Verification items for the finished model (mm, model axes). Face numbers are marked on the shaded views. A direction names the side the tool comes from. Give positions to 0.01 mm unless a question says otherwise; leave off trailing zeros. Order: outer loops, then holes, each group sorted by start corner. A loop starts at its lowest first (then second) coordinate and runs counter-clockwise, first axis right, second up. Notation, with made-up numbers: (65, -19) -> (77, -19) arc R36 ccw to (77, 16) -> close; hole circle Ø10 at (11, 72.25). An arc over 180 degrees is marked (long way). Return JSON: item names as keys, results as strings. Group by question number.
(1) Depth check by flat-ended pin: pin 1 Ø1 at (x, z) = (1, 2.5) entering from -Y; pin 2 Ø5 at (y, z) = (0.5, -9) entering from +X; pin 3 Ø2 at (x, z) = (-1, -8.5) entering from +Y. Enter the tip coordinate at first touch or a pass-through.
(2) Cross-section at B-B on z = -11.5. Enter the section's corners in (x, y), then the cut area to 3 significant figures.
(3) Thickness scan on line 1 along Z through (x, y) = (2.25, -2.25); line 2 along X through (y, z) = (1.75, -12.75); line 3 along Z through (x, y) = (0.25, -0.5). Record the ranges inside material, lowest first.
(4) Release check for a two-part mould opening along X. For the marked faces 3, 4 and 5 record: pulls with the +X half, pulls with the -X half, needs draft (parallel to the pull), parting line crosses it, or undercut.
(5) Tool access check on the marked faces 1 and 2. Record the directions out of +Z, -Z, +X, -X, +Y, -Y that give a thin tool (end or side, any length) a straight path to the whole face; none if there is none.
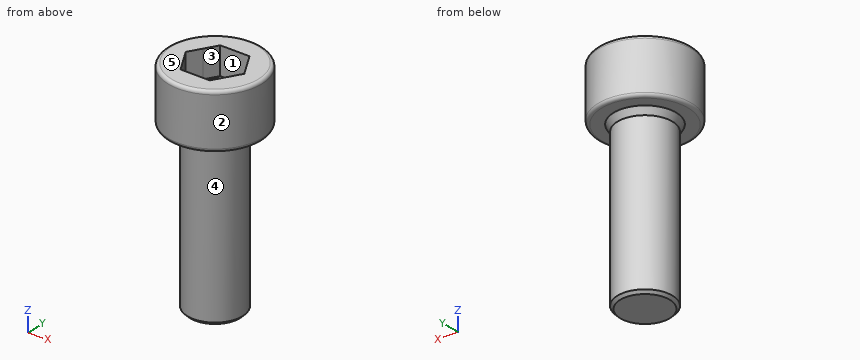
Solid Edge part; units mm, degrees
sketch "Sketch1" plane through (0, 0, 0) normal (0, -1, 0) x (1, 0, 0)
  line L0 (4.25, 5) -> (4.25, 0)
  line L1 (4.25, 0) -> (2.85, 0)
  line L2 (2.85, 0) -> (2.5, -0.6062)
  line L3 (2.5, -0.6062) -> (2.5, -15)
  line L4 (2.5, -15) -> (0, -15)
  line L5 (2.3, 2.5) -> (0, 1.1721)
  line L6 (2.3, 5) -> (2.3, 2.5)
  line L7 (4.25, 5) -> (2.3, 5)
revolve "RevolvedProtrusion1" add sketch "Sketch1" angle 360 about axis through (0, 0, -6) along (0, 0, 1)
cosmetic_thread "Thread1"
chamfer "chamfer" distance 0.25 angle 45 1 edges at (-2.5, 0, -15)
fillet "head_roundings" radius 0.3 2 edges at (-4.25, 0, 0) (-4.25, 0, 5)
sketch "Sketch2" plane through (0, 0, 5) normal (0, 0, 1) x (0, 1, 0)
  line L0 (-2.3, 1.3279) -> (-2.3, -1.3279)
  line L1 (0, -2.6558) -> (-2.3, -1.3279)
  line L2 (2.3, -1.3279) -> (0, -2.6558)
  line L3 (2.3, 1.3279) -> (2.3, -1.3279)
  line L4 (0, 2.6558) -> (2.3, 1.3279)
  line L5 (-2.3, 1.3279) -> (0, 2.6558)
extrude "Cutout1" cut sketch "Sketch2" against normal up to vertex (2.5 mm away)
properties part number "STD-DIN912-M5x15" material "Galvanized steel"
Verdict:
{
 "1": {"pin 1": "y = -4.22", "pin 2": "x = 2.5", "pin 3": "y = 2.5"},
 "2": {"outline": "circle Ø5 at (0, 0)", "area": "19.6 mm²"},
 "3": {"line 1": "0 to 5", "line 2": "-1.79 to 1.79", "line 3": "-15 to 1.49"},
 "4": {"face 3": "undercut", "face 4": "parting line crosses it", "face 5": "needs draft"},
 "5": {"face 1": "+Z", "face 2": "+Z, -Z"}
}
